Work out the finished part from the listing and answer in its coordinate system (mm). Face numbers are marked on the shaded views. A direction names the side the tool comes from. Coordinates: 2 decimals unless noted, no trailing zeros. Order: outer loops, then holes, each group sorted by start corner. A loop starts at its lowest first (then second) coordinate and runs counter-clockwise, first axis right, second up. Notation, with made-up numbers: M 18.5,13.25 L 42.5,13.25 A22 ccw 42.5,44.25 Z; hole C 76,36 d6. An arc over 180 degrees is marked long. Use a Markdown table: item, result.
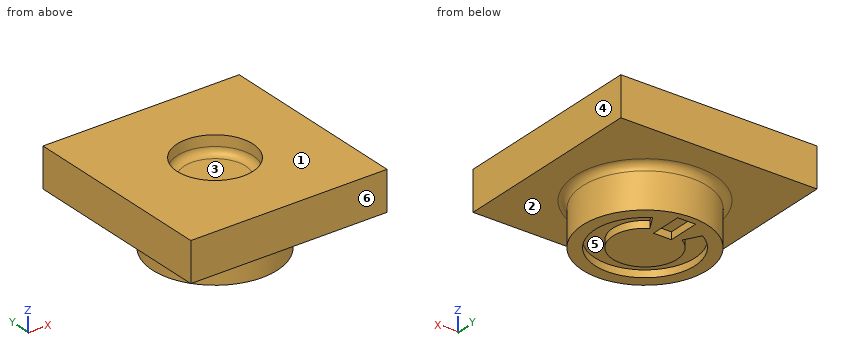
Autodesk Inventor part; units mm, degrees
ref_plane "YZ Plane" through (0, 0, 0) normal (1, 0, 0) x (0, 1, 0)
ref_plane "XZ Plane" through (0, 0, 0) normal (0, 1, 0) x (-1, 0, 0)
ref_plane "XY Plane" through (0, 0, 0) normal (0, 0, 1) x (1, 0, 0)
sketch "Sketch1" plane through (0, 0, 0) normal (0, 0, 1) x (1, 0, 0)
  line L0 (-4.7979, 3.7252) -> (6.2021, 3.7252)
  line L1 (6.2021, 3.7252) -> (6.2021, -7.2748)
  line L2 (6.2021, -7.2748) -> (-4.7979, -7.2748)
  line L3 (-4.7979, -7.2748) -> (-4.7979, 3.7252)
  circle A0 centre (0.7021, -1.7748) radius 3.5
  point P0 (0, 0)
  dimension "d0" = 11
  dimension "d1" = 11
  dimension "d2" = 7
extrude "Base" add sketch "Sketch1" along normal blind 2.2 contours L0 L1 L2 L3 | A0
extrude "Button" add sketch "Sketch1" against normal blind 2.4 contours A0
sketch "Sketch2" plane through (0, 0, 2.2) normal (0, 0, 1) x (1, 0, 0)
  circle A0 centre (0.7021, -1.7748) radius 2.125
  line L0 (6.2021, 3.7252) -> (-4.7979, 3.7252)
  line L1 (-4.7979, 3.7252) -> (-4.7979, -7.2748)
  point P0 (0, 0)
  dimension "d7" = 4.25
  dimension "d8" = 5.5
  dimension "d9" = 5.5
extrude "Tact switch button cutout" cut sketch "Sketch2" against normal blind 1
fillet "Cutout fillet" radius 0.4 1 edges at (-1.4229, -1.7748, 1.2)
fillet "Fillet2" radius 0.4 1 edges at (-2.7979, -1.7748, 0)
sketch "Sketch3" plane through (0.7021, -1.7748, -2.4) normal (0, 0, -1) x (-1, 0, 0)
  arc A0 (-1.4, 2.4249) -> (1.4, 2.4249) centre (0, 0) ccw
  line L0 (0, 0) -> (-1.4, 2.4249) construction
  line L1 (0, 0) -> (1.4, 2.4249) construction
  arc A1 (-0.9, 1.5588) -> (0.9, 1.5588) centre (0, 0) ccw
  line L2 (0, 0) -> (-0.9, 1.5588) construction
  line L3 (0, 0) -> (0.9, 1.5588) construction
  line L4 (-5.5, 5.5) -> (-5.5, -5.5)
  line L5 (5.5, 5.5) -> (-5.5, 5.5)
  line L6 (-1.4, 2.4249) -> (-0.9, 1.5588)
  line L7 (0.9, 1.5588) -> (1.4, 2.4249)
  line L8 (5.5, -5.5) -> (5.5, 5.5)
  line L9 (-0.5, 3.1) -> (0.5, 3.1)
  line L10 (0.5, 3.1) -> (0.5, 1.3)
  line L11 (0.5, 1.3) -> (-0.5, 1.3)
  line L12 (-0.5, 1.3) -> (-0.5, 3.1)
  point P0 (0.7021, 1.7748)
  dimension "d17" = 2.8
  dimension "d18" = 60
  dimension "d19" = 1.8
  dimension "d20" = 60
  dimension "d21" = 5.5
  dimension "d22" = 5.5
  dimension "d23" = 30
  dimension "d24" = 1
  dimension "d25" = 0.5
  dimension "d26" = 1.8
  dimension "d27" = 1.3
extrude "Power symbol" cut sketch "Sketch3" against normal blind 0.4
equation "\"d18\" = d20"
equation "\"d23\" = 0.5 * d20"
equation "\"d25\" = 0.5 * d24"
properties part number "power button"
(1) Given P1, Ø1.7, axis at x = 0, y = -2.5, coming from the +Z side; P2, Ø2, axis at x = 4, y = 2, coming from the -Z side, each flat-ended and moving along its own axis, determine where each tip first touches the part or whether it passes through.
Conclusion:
| item | result |
|---|---|
| P1 | z = 1.22 |
| P2 | z = 0 |
(2) Determine the mould class of the marked faces 3, 4, 5 and 6 for opening direction Y: pulls with the +Y half, pulls with the -Y half, needs draft (parallel to the pull), parting line crosses it, or undercut.
Conclusion:
| item | result |
|---|---|
| face 3 | undercut |
| face 4 | needs draft |
| face 5 | undercut |
| face 6 | pulls with the -Y half |
(3) A cutting plane is placed at B-B (z = -0.75). Determine the outline of the cut face in (x, y), then the cut area to 3 significant figures.
Conclusion:
| item | result |
|---|---|
| outline | C 0.7,-1.77 d7 |
| area | 38.5 mm2 |
(4) A cutting plane is placed at A-A (x = 5.25). Determine the outline of the cut face in (y, z).
Conclusion:
| item | result |
|---|---|
| outline | M -7.27,0 L 3.73,0 L 3.73,2.2 L -7.27,2.2 Z |
(5) Straight lines are drawn through the part: L1, parallel to X at y = 0, z = 1.8; L2, parallel to Z at x = -2, y = -1.5; L3, parallel to Z at x = 5, y = -3.25. For each, find the intervals that lie inside material, in ascending order.
Conclusion:
| item | result |
|---|---|
| L1 | -4.8 to -0.47, 1.87 to 6.2 |
| L2 | -2 to 2.2 |
| L3 | 0 to 2.2 |
(6) Which of the six approach directions +Z, -Z, +X, -X, +Y, -Y give full straight-line access (tool end or side, diameter ignored) to the marked faces 1 and 2?
Conclusion:
| item | result |
|---|---|
| face 1 | +Z, +X, -X, +Y, -Y |
| face 2 | -Z |
